Model file for the job. Use its own axes, mm. A direction names the side the tool comes from. Coordinates: 2 decimals unless noted, no trailing zeros. Write each loop counter-clockwise with the first axis right and the second up, starting at its lowest first coordinate (ties: lowest second). Pieces come first, ordered by that corner, then holes. Notation, with made-up numbers: M 12,23 L 21,23 A13 ccw 21,44 Z; hole C 35,16.25 d9. An arc over 180 degrees is marked long. Put each result on its own line as item: value. Start each with the question number.
Q1. Pull direction X, two halves, no side cores. Call faces 4 (the flat face through (-54.7, 3, 0)), 5 (the flat face through (67, 3, 6.1)), 6 (the cylindrical face through (-2.6, 0.6, 4.8)): pulls with the +X half, pulls with the -X half, needs draft (parallel to the pull), parting line crosses it, or undercut.
Q2. Cut at A-A (y = 6.75). Write the cut outline in (x, z) (3 decimals).
Q3. Drill centre lines: line 1 along X through (y, z) = (0.3, -6.2); line 2 along X through (y, z) = (3.25, -2.5); line 3 along Z through (x, y) = (-77, 0.55). Where is each one in solid material? Low to high.
Q4. Drop flat-ended pins along their axis: pin 1 (1.1 mm diameter, centred on y = 3, z = 2.5, fed in from +X); pin 2 (5 mm diameter, centred on y = 4.5, z = 0.5, fed in from -X); pin 3 (4 mm diameter, centred on x = -13.5, y = 3.5, fed in from -Z); pin 4 (1.5 mm diameter, centred on x = 77, z = -6.2, fed in from -Y). Give the stop position or say it passes through.
Q5. Which spindle directions (+Z, -Z, +X, -X, +Y, -Y) get a long thin tool onto all of the face, cutting with end or side? Do faces 1 (the flat face through (6, 3, -6.1)), 2 (the flat face through (6, 3, 6.1)), 3 (the flat face through (68.8, 3, 0)). Say none if no direction does.
Q6. Cut at B-B (z = -1.25). Write the cut outline in (x, y).
Q7. Cut at C-C (x = -22.5). Write the cut outline in (y, z).
Autodesk Inventor part; units mm, degrees
ref_plane "YZ Plane" through (0, 0, 0) normal (1, 0, 0) x (0, 1, 0)
ref_plane "XZ Plane" through (0, 0, 0) normal (0, 1, 0) x (-1, 0, 0)
ref_plane "XY Plane" through (0, 0, 0) normal (0, 0, 1) x (1, 0, 0)
sketch "Sketch1" plane through (0, 0, 0) normal (0, 1, 0) x (-1, 0, 0)
  line L0 (79, -8) -> (-79, -8)
  line L1 (-79, -8) -> (-79, 8)
  line L2 (79, 8) -> (79, -8)
  line L3 (79, -8) -> (-79, 8) construction
  line L4 (-79, -8) -> (79, 8) construction
  arc A0 (-1.6, 8) -> (6.6, 8) centre (2.5, 9.0266) ccw
  line L5 (0, -8) -> (0, 2.5887)
  line L6 (2.5, 9.0266) -> (2.5, 15.2917) construction
  line L7 (7.7992, 4.8) -> (-2.6665, 4.8) construction
  line L8 (-79, 8) -> (-1.6, 8)
  line L9 (6.6, 8) -> (79, 8)
  point P0 (0, 0)
  dimension "d0" = 158
  dimension "d1" = 16
  dimension "d2" = 76.5
  dimension "d3" = 8.2
  dimension "d5" = 3.2
extrude "Extrusion1" add sketch "Sketch1" along normal blind 1.3
sketch "Sketch2" plane through (0, 1.3, 0) normal (0, 1, 0) x (1, 0, 0)
  line L0 (79, 8) -> (-79, 8)
  line L1 (-79, 8) -> (-79, -8)
  line L2 (-79, -8) -> (-6.6, -8)
  arc A0 (1.6, -8) -> (-6.6, -8) centre (-2.5, -9.0266) ccw
  line L3 (1.6, -8) -> (79, -8)
  line L4 (79, -8) -> (79, 8)
  line L5 (-77, 6.2) -> (77, 6.2) construction
  line L6 (19.5, 6.2) -> (19.5, -6.2) construction
  point P0 (0, 0)
  dimension "d8" = 154
  dimension "d9" = 1.8
  dimension "d10" = 1.8
  dimension "d11" = 57.5
  dimension "d19" = 2
  dimension "d20" = 2
  dimension "d47" = 59.5
hole "Hole1" at (-77, 1.3, -6.2) at (77, 1.3, -6.2) at (19.5, 1.3, -6.2) at (19.5, 1.3, 6.2) direction (0, -1, 0) diameter 1.9 end through all
sketch "Sketch3" plane through (0, 1.3, 0) normal (0, 1, 0) x (1, 0, 0)
  line L0 (-16.35, 7.5) -> (-6.5, 7.5)
  line L1 (-6.5, 7.5) -> (-6.5, 5.5)
  line L2 (-6.5, 5.5) -> (-16.35, 5.5)
  line L3 (-16.35, 5.5) -> (-16.35, 7.5)
  line L4 (-16.35, 7.5) -> (-6.5, 5.5) construction
  line L5 (-6.5, 7.5) -> (-16.35, 5.5) construction
  line L6 (79, 8) -> (-79, 8)
  line L7 (-79, 8) -> (-79, -8)
  line L8 (-54.7, -5.85) -> (-51.7, -5.85)
  line L9 (-51.7, -5.85) -> (-51.7, 5.85)
  line L10 (-51.7, 5.85) -> (-54.7, 5.85)
  line L11 (-54.7, 5.85) -> (-54.7, -5.85)
  line L12 (-54.7, -5.85) -> (-51.7, 5.85) construction
  line L13 (-51.7, -5.85) -> (-54.7, 5.85) construction
  line L14 (4.6, -6.1) -> (7.4, -6.1)
  line L15 (7.4, -6.1) -> (7.4, 6.1)
  line L16 (7.4, 6.1) -> (4.6, 6.1)
  line L17 (4.6, 6.1) -> (4.6, -6.1)
  line L18 (4.6, -6.1) -> (7.4, 6.1) construction
  line L19 (7.4, -6.1) -> (4.6, 6.1) construction
  line L20 (66, -6.1) -> (68.8, -6.1)
  line L21 (68.8, -6.1) -> (68.8, 6.1)
  line L22 (68.8, 6.1) -> (66, 6.1)
  line L23 (66, 6.1) -> (66, -6.1)
  line L24 (66, -6.1) -> (68.8, 6.1) construction
  line L25 (68.8, -6.1) -> (66, 6.1) construction
  line L26 (6, 0) -> (67.4, 0) construction
  line L27 (79, -8) -> (79, 8)
  point P0 (0, 0)
  point P1 (-11.425, 6.5)
  point P2 (-53.2, 0)
  point P3 (-53.2, 0)
  dimension "d21" = 9.85
  dimension "d22" = 2
  dimension "d23" = 0.5
  dimension "d24" = 72.5
  dimension "d25" = 3
  dimension "d26" = 11.7
  dimension "d27" = 2.8
  dimension "d28" = 12.2
  dimension "d29" = 12.2
  dimension "d30" = 2.8
  dimension "d31" = 74.4
  dimension "d32" = 13
  dimension "d33" = 27.3
extrude "Extrusion2" add sketch "Sketch3" along normal blind 3.6
sketch "Sketch4" plane through (0, 4.9, 0) normal (0, 1, 0) x (1, 0, 0)
  line L0 (-6.5, 7.5) -> (-16.35, 7.5)
  line L1 (-16.35, 7.5) -> (-16.35, 5.5)
  line L2 (-16.35, 5.5) -> (-6.5, 5.5)
  line L3 (-6.5, 5.5) -> (-6.5, 7.5)
  line L4 (-16.35, 6.5) -> (-6.5, 6.5) construction
  line L5 (-6.5, 7.5) -> (-6.5, 5.5)
  circle A0 centre (-15.375, 6.5) radius 0.25
  circle A1 centre (-7.475, 6.5) radius 0.25
  circle A2 centre (-13.4, 6.5) radius 0.25
  circle A3 centre (-11.425, 6.5) radius 0.25
  circle A4 centre (-9.45, 6.5) radius 0.25
  line L6 (-6.5, 5.5) -> (-16.35, 5.5)
  line L7 (-11.425, 5.5) -> (-11.425, 4.6298) construction
  point P0 (0, 0)
  dimension "d36" = 0.5
  dimension "d37" = 0.5
  dimension "d38" = 7.9
  dimension "d39" = 0.5
  dimension "d40" = 0.5
  dimension "d41" = 0.5
  dimension "d42" = 1.975
  dimension "d43" = 1.975
  dimension "d44" = 1.975
extrude "Extrusion3" add sketch "Sketch4" along normal blind 3.6 contours A0 | A1 | A2 | A3 | A4
equation "\"d10\" = d9"
equation "\"d29\" = d28"
equation "\"d30\" = d27"
equation "\"d42\" = 0.25 * d38"
equation "\"d43\" = d42"
equation "\"d44\" = d43"
properties part number "xtion_mainboard"
Computed values:
1. face 4: pulls with the -X half
1. face 5: needs draft
1. face 6: undercut
2. outline: C -15.375,-6.5 d0.5; C -13.4,-6.5 d0.5; C -11.425,-6.5 d0.5; C -9.45,-6.5 d0.5; C -7.475,-6.5 d0.5
3. line 1: -79 to -77.95, -76.05 to 18.55, 20.45 to 76.05, 77.95 to 79
3. line 2: -54.7 to -51.7, 4.6 to 7.4, 66 to 68.8
3. line 3: -8 to -7.15, -5.25 to 8
4. pin 1: x = 68.8
4. pin 2: x = -54.7
4. pin 3: z = -7.5
4. pin 4: through
5. face 1: -Z, +X, +Y
5. face 2: +Z, +X, -X, +Y
5. face 3: +Z, -Z, +X, +Y
6. outline: M -79,0 L 79,0 L 79,1.3 L 68.8,1.3 L 68.8,4.9 L 66,4.9 L 66,1.3 L 7.4,1.3 L 7.4,4.9 L 4.6,4.9 L 4.6,1.3 L -51.7,1.3 L -51.7,4.9 L -54.7,4.9 L -54.7,1.3 L -79,1.3 Z
7. outline: M 0,-8 L 1.3,-8 L 1.3,8 L 0,8 Z
